Can you work these out from the model? Positions are in its coordinate system, mm. Face numbers are marked on the shaded views. A direction names the side the tool comes from. Give positions to 0.01 mm unless a question says otherwise; leave off trailing zeros. Loops run counter-clockwise (first coordinate to the right, second up) from the corner with the lowest first, then second, coordinate; pieces in that order, holes last. Notation, with made-up numbers: (37, 89.25) - (85, 89.25) arc R20 cw to (85, 126.25) - close; hole circle Ø11 at (32.5, -13.75). An arc over 180 degrees is marked (long way). Answer in a Markdown table with one row per item.
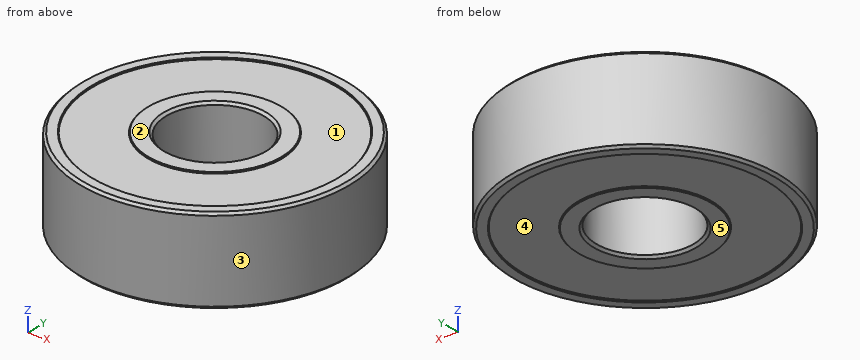
from build123d import *

# Parameters (mm, degrees)
SKETCH1_W                = 11
SKETCH1_H                = 7
SKETCH2_R                = 10.05
CUT_EXTRUDE1_DEPTH       = 0.05
CUT_EXTRUDE1_DRAFT       = -45
SKETCH3_R                = 10
CUT_EXTRUDE2_DEPTH       = 0.05
SKETCH4_R                = 5.5
BOSS_EXTRUDE1_DEPTH      = 0.05
SKETCH5_R                = 5.5
BOSS_EXTRUDE2_DEPTH      = 0.05
BOSS_EXTRUDE2_TAPER      = 45
SKETCH6_R                = 10.05
CUT_EXTRUDE3_DEPTH       = 0.05
CUT_EXTRUDE3_DRAFT       = -45
CUT_EXTRUDE4_START       = -0.05
SKETCH7_R                = 10
CUT_EXTRUDE4_DEPTH       = 0.05
F_8_0_8_DIAMETER_HOLE1_D = 8
CHAMFER1_SIZE            = 0.2


with BuildPart() as part:
    # Sketch1 → Revolve1 (revolve)
    with BuildSketch(Plane.XZ, mode=Mode.PRIVATE) as revolve1_sk:
        with Locations((5.5, 3.5)):
            Rectangle(SKETCH1_W, SKETCH1_H)
    revolve(revolve1_sk.sketch.rotate(Axis((0, 0, 7), (0, 0, -1)), 180), axis=Axis((0, 0, 7), (0, 0, -1)))


with BuildPart() as cut_extrude1_tool:
    # Sketch2 → Cut-Extrude1 (with draft: the straight prism first)
    with BuildSketch(Plane(origin=(0, 0, 0), x_dir=(-1, 0, 0), z_dir=(0, 0, -1))):
        Circle(SKETCH2_R)
    extrude(amount=-CUT_EXTRUDE1_DEPTH)
    # Cut-Extrude1: the draft: its side faces are tilted about the plane it starts from
    cut_extrude1_sides = [cut_extrude1_tool.faces().sort_by_distance(p)[0] for p in [
        (10.05, 0, 0.025),
    ]]
    draft(cut_extrude1_sides, Plane(origin=(0, 0, 0), x_dir=(-1, 0, 0), z_dir=(0, 0, -1)), CUT_EXTRUDE1_DRAFT)


with BuildPart() as part_1:
    add(part.part)

    # Cut-Extrude1: cut by cut_extrude1_tool
    add(cut_extrude1_tool.part, mode=Mode.SUBTRACT)

    # Sketch3 → Cut-Extrude2 (cut)
    with BuildSketch(Plane(origin=(0, 0, 0.05), x_dir=(-1, 0, 0), z_dir=(0, 0, -1))):
        with Locations(Location((0, 0, 0), (0, 0, 180))):
            Circle(SKETCH3_R)
    extrude(amount=-CUT_EXTRUDE2_DEPTH, mode=Mode.SUBTRACT)

    # Sketch4 → Boss-Extrude1 (add)
    with BuildSketch(Plane(origin=(0, 0, 0.1), x_dir=(-1, 0, 0), z_dir=(0, 0, -1))):
        with Locations(Location((0, 0, 0), (0, 0, 180))):
            Circle(SKETCH4_R)
    extrude(amount=BOSS_EXTRUDE1_DEPTH)

    # Sketch5 → Boss-Extrude2 (add)
    with BuildSketch(Plane(origin=(0, 0, 0.05), x_dir=(-1, 0, 0), z_dir=(0, 0, -1))):
        with Locations(Location((0, 0, 0), (0, 0, 180))):
            Circle(SKETCH5_R)
    extrude(amount=BOSS_EXTRUDE2_DEPTH, taper=BOSS_EXTRUDE2_TAPER)


with BuildPart() as cut_extrude3_tool:
    # Sketch6 → Cut-Extrude3 (with draft: the straight prism first)
    with BuildSketch(Plane.XY.offset(7)):
        Circle(SKETCH6_R)
    extrude(amount=-CUT_EXTRUDE3_DEPTH)
    # Cut-Extrude3: the draft: its side faces are tilted about the plane it starts from
    cut_extrude3_sides = [cut_extrude3_tool.faces().sort_by_distance(p)[0] for p in [
        (-10.05, 0, 6.975),
    ]]
    draft(cut_extrude3_sides, Plane.XY.offset(7), CUT_EXTRUDE3_DRAFT)


with BuildPart() as part_2:
    add(part_1.part)

    # Cut-Extrude3: cut by cut_extrude3_tool
    add(cut_extrude3_tool.part, mode=Mode.SUBTRACT)

    # Sketch7 → Cut-Extrude4 (cut)
    with BuildSketch(Plane.XY.offset(6.95).offset(CUT_EXTRUDE4_START)):
        Circle(SKETCH7_R)
    extrude(amount=CUT_EXTRUDE4_DEPTH, mode=Mode.SUBTRACT)

    # Sketch8 → Revolve2 (revolve)
    with BuildSketch(Plane(origin=(0, 0, 0), x_dir=(1, 0, 0), z_dir=(0, 1, 0))):
        Polygon((5.5, -6.9), (0, -6.9), (0, -7), (5.45, -7), (5.5, -6.95), align=None)
    revolve(axis=Axis((0, 0, 6.9), (0, 0, 1)))

    # Ø8.0 (8) Diameter Hole1 (through all)
    with Locations(Plane.XY.offset(7)):
        with Locations((0, 0)):
            Hole(F_8_0_8_DIAMETER_HOLE1_D / 2)

    # Chamfer1
    chamfer1_edges = [part_2.edges().sort_by_distance(p)[0] for p in [
        (11, 0, 0),
        (4, 0, 7),
        (4, 0, 0),
        (11, 0, 7),
    ]]
    chamfer(chamfer1_edges, length=CHAMFER1_SIZE)


solid = part_2.part
Q1. For pin 1 (1.5 mm diameter, centred on x = 3, z = 2, fed in from +Y); pin 2 (2 mm diameter, centred on y = -2, z = 6, fed in from -X); pin 3 (2 mm diameter, centred on x = 4, z = 1, fed in from -Y), each with a flat end and sliding along its axis, tell me the tip position at first contact or that it passes through.
Checked values:
| item | result |
|---|---|
| pin 1 | stops at y = 10.77 |
| pin 2 | stops at x = -10.95 |
| pin 3 | stops at y = -10.58 |
Q2. If we mould it in two halves opening along X, with no side actions, what happens to the marked faces 3, 4 and 5? For each: released by +X, released by -X, zero draft, split by the parting line, or undercut.
Checked values:
| item | result |
|---|---|
| face 3 | split by the parting line |
| face 4 | undercut |
| face 5 | zero draft |
Q3. Imagine slicing it at A-A, the plane z = 3. Write out the boundary of the cut face in (x, y).
Checked values:
| item | result |
|---|---|
| outline | circle Ø22 at (0, 0); hole circle Ø8 at (0, 0) |
Q4. If I drill on line 1 (Y direction, x = 0, z = 2.25); line 2 (Z direction, x = 0.5, y = 7.5); line 3 (X direction, y = 2.5, z = 5.5), over which ranges is the centre line in solid material (lowest first)? Write a range as [from, to].
Checked values:
| item | result |
|---|---|
| line 1 | y = [-11, -4], [4, 11] |
| line 2 | z = [0.1, 6.9] |
| line 3 | x = [-10.71, -3.12], [3.12, 10.71] |
Q5. On a 3-axis mill with a long thin cutter (end or side, diameter ignored), from which of +Z, -Z, +X, -X, +Y, -Y can I reach the whole of each face in a straight line? I mean the marked faces 1 and 2. Say none if no direction works.
Checked values:
| item | result |
|---|---|
| face 1 | +Z |
| face 2 | +Z, +X, -X, +Y, -Y |
